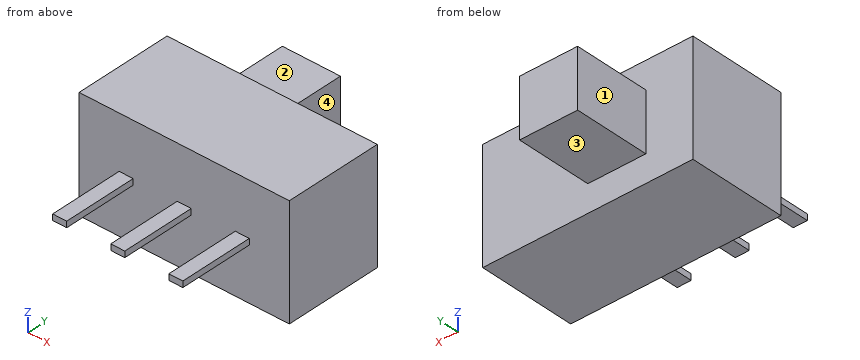
```python
from build123d import *

# Parameters (mm, degrees)
ESQUISSE1_W        = 10.5
ESQUISSE1_H        = 5.6
BOSS_EXTRU_1_DEPTH = 4.9
ESQUISSE2_W        = 2.9
ESQUISSE2_H        = 2.9
BOSS_EXTRU_2_DEPTH = 3.8
ESQUISSE3_W        = 0.7
ESQUISSE3_H        = 0.3
BOSS_EXTRU_3_DEPTH = 3.7


with BuildPart() as part:
    # Esquisse1 → Boss.-Extru.1 (new body)
    with BuildSketch(Plane(origin=(0, 0, 0), x_dir=(1, 0, 0), z_dir=(0, 1, 0))):
        Rectangle(ESQUISSE1_W, ESQUISSE1_H)
    extrude(amount=BOSS_EXTRU_1_DEPTH)

    # Esquisse2 → Boss.-Extru.2 (add)
    with BuildSketch(Plane(origin=(0, 4.9, 0), x_dir=(1, 0, 0), z_dir=(0, 1, 0))):
        with Locations((-1.45, 0)):
            Rectangle(ESQUISSE2_W, ESQUISSE2_H)
    extrude(amount=BOSS_EXTRU_2_DEPTH)

    # Esquisse3 → Boss.-Extru.3 (add)
    with BuildSketch(Plane.XZ):
        Rectangle(ESQUISSE3_W, ESQUISSE3_H)
        with Locations((2.9, 0)):
            Rectangle(ESQUISSE3_W, ESQUISSE3_H)
        with Locations((-2.9, 0)):
            Rectangle(ESQUISSE3_W, ESQUISSE3_H)
    extrude(amount=BOSS_EXTRU_3_DEPTH)


solid = part.part
```
Read the model definition and answer for the solid it produces. Units are mm, in the model's axes. Face numbers are marked on the shaded views. A direction names the side the tool comes from. Give positions to 0.01 mm unless a question says otherwise; leave off trailing zeros. Loops run counter-clockwise (first coordinate to the right, second up) from the corner with the lowest first, then second, coordinate; pieces in that order, holes last.
Item 1: The part is cut by section C-C (x = 3). Write down the section's boundary in (y, z), and give its area (4 significant figures).
Item 2: Each of these flat-tipped pins is pushed along its axis until it touches: pin 1 Ø0.6 at (x, y) = (0, -1) entering from +Z; pin 2 Ø1.4 at (y, z) = (6.5, -0.5) entering from +X; pin 3 Ø0.9 at (x, y) = (-1.5, 6.5) entering from -Z. Where does it stop, or does it pass through?
Item 3: The part is cut by section D-D (y = 7). Write down the section's boundary in (x, z), and give its area (3 significant figures).
Item 4: Find the intervals of material crossed by line 1 along X through (y, z) = (6.75, -0.9); line 2 along Y through (x, z) = (1.5, 1.75); line 3 along Z through (x, y) = (-0.25, 7.5), in increasing order.
Item 5: For the marked faces 1, 2, 3 and 4, determine the directions among +Z, -Z, +X, -X, +Y, -Y from which every point of the face is accessible in a straight line to the end or side of a thin tool.
Item 6: The part is cut by section A-A (y = -0.5). Write down the section's boundary in (x, z), and give its area (3 significant figures).
Item 7: The part is cut by section B-B (z = 0.5). Write down the section's boundary in (x, y), and give its area (3 significant figures).
Taken from the geometry:
1. outline: (-3.7, -0.15) - (0, -0.15) - (0, -2.8) - (4.9, -2.8) - (4.9, 2.8) - (0, 2.8) - (0, 0.15) - (-3.7, 0.15) - close
1. area: 28.55 mm2
2. pin 1: stops at z = 0.15
2. pin 2: stops at x = 0
2. pin 3: stops at z = -1.45
3. outline: (-2.9, -1.45) - (0, -1.45) - (0, 1.45) - (-2.9, 1.45) - close
3. area: 8.41 mm2
4. line 1: x = -2.9 to 0
4. line 2: y = 0 to 4.9
4. line 3: z = -1.45 to 1.45
5. face 1: +Z, -Z, -X, +Y
5. face 2: +Z, +X, -X, +Y
5. face 3: -Z, +X, -X, +Y
5. face 4: +Z, -Z, +X, +Y
6. outline: (-3.25, -0.15) - (-2.55, -0.15) - (-2.55, 0.15) - (-3.25, 0.15) - close; (-0.35, -0.15) - (0.35, -0.15) - (0.35, 0.15) - (-0.35, 0.15) - close; (2.55, -0.15) - (3.25, -0.15) - (3.25, 0.15) - (2.55, 0.15) - close
6. area: 0.630 mm2
7. outline: (-5.25, 0) - (5.25, 0) - (5.25, 4.9) - (0, 4.9) - (0, 8.7) - (-2.9, 8.7) - (-2.9, 4.9) - (-5.25, 4.9) - close
7. area: 62.5 mm2
